Work out the finished part from the listing and answer in its coordinate system (mm). A direction names the side the tool comes from. Round coordinates to 2 decimals unless told otherwise and drop trailing zeros. Loops run counter-clockwise (first coordinate to the right, second up) from the corner with the lowest first, then second, coordinate; pieces in that order, holes last.
from build123d import *

# Parameters (mm, degrees)
F0_R     = 30
F1_DEPTH = 4
F3_DEPTH = 8
F4_R     = 2
F5_DEPTH = 12
F6_R     = 13.5
F7_DEPTH = 50


with BuildPart() as f1:
    # F0 (on Top) → F1 (new body)
    with BuildSketch(Plane.XY):
        Circle(F0_R)
    extrude(amount=-F1_DEPTH)

    # F2 (on face) → F3 (join)
    with BuildSketch(Plane(origin=(0, 0, -4), x_dir=(1, 0, 0), z_dir=(0, 0, -1))):
        Polygon((-40, 31), (-40, -33), (40, -33), (40, 31), (0, 31), align=None)
        with BuildLine():
            ThreePointArc((30, 0), (-21.2132034356, -21.2132034356), (0, 30))
            ThreePointArc((0, 30), (21.2132034356, 21.2132034356), (30, 0))
        make_face(mode=Mode.SUBTRACT)
        with BuildLine():
            ThreePointArc((30, 0), (21.2132034356, 21.2132034356), (0, 30))
            ThreePointArc((0, 30), (-21.2132034356, -21.2132034356), (30, 0))
        make_face()
    extrude(amount=F3_DEPTH)

    # F4 (on face) → F5 (join)
    with BuildSketch(Plane.XY.offset(-4)):
        with Locations((-32, -17)):
            Circle(F4_R)
        with Locations((32, -17)):
            Circle(F4_R)
    extrude(amount=F5_DEPTH)

    # F6 (on face) → F7 (join)
    with BuildSketch(Plane.XY.offset(-4)):
        with Locations((0, -16.5)):
            Circle(F6_R)
    extrude(amount=F7_DEPTH)


solid = f1.part
Item 1: Section A-A, the plane y = 18 is taken. Give the vertices of the cut face in (x, z).
Item 2: Section D-D, the plane y = -21 is taken. Give the vertices of the cut face in (x, z).
Item 3: Straight lines are drawn through the part: line 1 (Z direction, x = -22, y = 22); line 2 (Z direction, x = 13, y = 18); line 3 (X direction, y = -23.5, z = 35). For each, find the intervals that lie inside material, in ascending order.
Item 4: Determine the mould class of faces 1 (the face through (-40, 1, -8)), 2 (the face through (-30.092, -16.399, 1.916)), 3 (the face through (40, 1, -8)) for opening direction X: pulls with the +X half, pulls with the -X half, needs draft (parallel to the pull), parting line crosses it, or undercut.
Item 5: Section C-C, the plane z = 15.5 is taken. Give the vertices of the cut face in (x, y).
Item 6: For faces 4 (the face through (-32, -17, 8)), 5 (the face through (32, -17, 8)), 6 (the face through (33.908, -16.399, 1.916)), determine the directions among +Z, -Z, +X, -X, +Y, -Y from which every point of the face is accessible in a straight line to the end or side of a thin tool.
Item 7: Section B-B, the plane x = 32 is taken. Give the vertices of the cut face in (y, z).
Item 8: Each of these flat-tipped pins is pushed along its axis until it touches: P1, Ø1.2, axis at x = 31.5, y = -16.5, coming from the +Z side; P2, Ø6, axis at x = -15, z = 22.5, coming from the -Y side; P3, Ø4, axis at y = -23, z = 17, coming from the -X side; P4, Ø19, axis at x = -3.5, y = 5.5, coming from the +Z side. Where does it stop, or does it pass through?
Answer below:
1. outline: (-40, -12) - (40, -12) - (40, -4) - (24, -4) - (24, 0) - (-24, 0) - (-24, -4) - (-40, -4) - close
2. outline: (-40, -12) - (40, -12) - (40, -4) - (21.42, -4) - (21.42, 0) - (12.73, 0) - (12.73, 46) - (-12.73, 46) - (-12.73, 0) - (-21.42, 0) - (-21.42, -4) - (-40, -4) - close
3. line 1: z = -12 to -4
3. line 2: z = -12 to 0
3. line 3: x = -11.54 to 11.54
4. face 1: pulls with the -X half
4. face 2: undercut
4. face 3: pulls with the +X half
5. outline: circle Ø27 at (0, -16.5)
6. face 4: +Z, -X, +Y, -Y
6. face 5: +Z, +X, +Y, -Y
6. face 6: +Z
7. outline: (-31, -12) - (33, -12) - (33, -4) - (-15, -4) - (-15, 8) - (-19, 8) - (-19, -4) - (-31, -4) - close
8. P1: stops at z = 8
8. P2: stops at y = -22.68
8. P3: stops at x = -12.73
8. P4: stops at z = 46
